Can you work these out from the model? Positions are in its coordinate system, mm. Face numbers are marked on the shaded views. A direction names the side the tool comes from. Round coordinates to 2 decimals unless told otherwise and drop trailing zeros. Loops run counter-clockwise (first coordinate to the right, second up) from the corner with the lowest first, then second, coordinate; pieces in that order, holes last. Notation, with made-up numbers: (47.5, 10.25) -> (66.5, 10.25) arc R22 ccw to (66.5, 44.25) -> close; hole circle Ø7 at (-22, 31). An arc over 180 degrees is marked (long way). Write item = value, one per line.
from build123d import *

# Parameters (mm, degrees)
F0_W     = 100
F0_H     = 100
F1_DEPTH = 50
F3_DEPTH = 100
F4_R     = 10
F5_DEPTH = 50
F7_DEPTH = 25
F8_W     = 80
F8_H     = 37.447
F9_DEPTH = 150


with BuildPart() as f1:
    # F0 (on Top) → F1 (new body)
    with BuildSketch(Plane.XY):
        with Locations((-7.640187, 1.520901)):
            Rectangle(F0_W, F0_H)
    extrude(amount=F1_DEPTH)

    # F2 (on face) → F3 (cut)
    with BuildSketch(Plane.XZ.offset(48.479099)):
        Polygon((0, 52.099957), (-27.144263, 52.099957), (-27.144263, 7.099957), (17.855737, 7.099957), (17.855737, 52.099957), align=None)
    extrude(amount=-F3_DEPTH, mode=Mode.SUBTRACT)

    # F4 (on face) → F5 (join)
    with BuildSketch(Plane(origin=(0, 0, 0), x_dir=(1, 0, 0), z_dir=(0, 0, -1))):
        with Locations((-57.640187, -51.520901)):
            Circle(F4_R)
        with Locations((-57.640187, 48.479099)):
            Circle(F4_R)
        with Locations((42.359813, 48.479099)):
            Circle(F4_R)
        with Locations((42.359813, -51.520901)):
            Circle(F4_R)
    extrude(amount=-F5_DEPTH)

    # F6 (on face) → F7 (cut)
    with BuildSketch(Plane(origin=(0, 0, 0), x_dir=(1, 0, 0), z_dir=(0, 0, -1))):
        Polygon((-14.585404, 10.162264), (-14.585404, -11.031568), (5.571128, -17.580822), (18.02855, -0.434652), (5.571128, 16.711519), align=None)
    extrude(amount=-F7_DEPTH, mode=Mode.SUBTRACT)

    # F8 (on face) → F9 (cut)
    with BuildSketch(Plane(origin=(-57.640187, 0, 0), x_dir=(0, -1, 0), z_dir=(-1, 0, 0))):
        with Locations((-1.520901, 31.2765)):
            Rectangle(F8_W, F8_H)
    extrude(amount=-F9_DEPTH, mode=Mode.SUBTRACT)


solid = f1.part
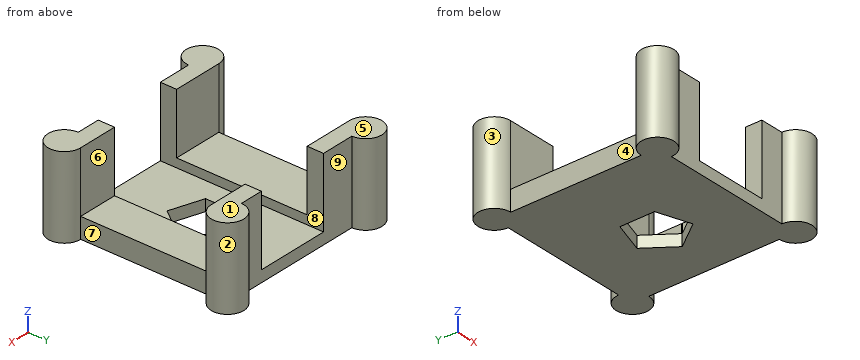
1. Suppose I cut it at A-A, the plane z = 10. List the corners of the cut face in (x, y) for me.
Entries:
outline = (-57.64, -38.48) arc R10 ccw (long way) to (-47.64, -48.48) -> (-27.14, -48.48) -> (-27.14, 51.52) -> (-47.64, 51.52) arc R10 ccw (long way) to (-57.64, 41.52) -> close; (17.86, -48.48) -> (32.36, -48.48) arc R10 ccw (long way) to (42.36, -38.48) -> (42.36, 41.52) arc R10 ccw (long way) to (32.36, 51.52) -> (17.86, 51.52) -> (17.86, 0.67) -> (18.03, 0.43) -> (17.86, 0.2) -> close
2. Suppose I cut it at D-D, the plane y = 38. List the corners of the cut face in (x, z) for me, and give its area (3 significant figures).
Entries:
outline = (-57.64, 0) -> (42.36, 0) -> (42.36, 12.55) -> (17.86, 12.55) -> (17.86, 7.1) -> (-27.14, 7.1) -> (-27.14, 12.55) -> (-57.64, 12.55) -> close
area = 1,010 mm²
3. We'd pull the mould along X, two halves only. Please class the marked faces 1, 2, 3 and 4: released by +X, released by -X, zero draft, split by the parting line, or undercut.
Entries:
face_1 = zero draft
face_2 = undercut
face_3 = undercut
face_4 = released by -X
4. For the marked faces 5, 6, 7, 8 and 9, which set-ups out of +Z, -Z, +X, -X, +Y, -Y let a thin tool reach every point of the face, with its end or its side?
Entries:
face_5 = +Z, +X, -X, +Y, -Y
face_6 = +Z, +X, -X
face_7 = +Z, -Z, +X
face_8 = +Z, +Y, -Y
face_9 = +Z, -Z, +Y
5. Suppose I cut it at B-B, the plane z = 17.5. List the corners of the cut face in (x, y) for me, and give its area (3 significant figures).
Entries:
outline = (-57.64, -38.48) arc R10 ccw (long way) to (-47.64, -48.48) -> (-27.14, -48.48) -> (-27.14, -38.48) -> close; (-57.64, 41.52) -> (-27.14, 41.52) -> (-27.14, 51.52) -> (-47.64, 51.52) arc R10 ccw (long way) to start; (17.86, -48.48) -> (32.36, -48.48) arc R10 ccw (long way) to (42.36, -38.48) -> (17.86, -38.48) -> close; (17.86, 41.52) -> (42.36, 41.52) arc R10 ccw (long way) to (32.36, 51.52) -> (17.86, 51.52) -> close
area = 2,040 mm²
6. I need wall thicknesses on line 1 (Y direction, x = -43.5, z = 38); line 2 (X direction, y = 37, z = 9.5); line 3 (Z direction, x = 12, y = -21.5). Which ranges of each line are inside material? Lowest first, please. Write a range as [from, to].
Entries:
line_1 = [-48.48, -38.48], [41.52, 51.52]
line_2 = [-57.64, -27.14], [17.86, 42.36]
line_3 = [0, 7.1]
7. I'm going to push flat-ended pins straight in: pin 1 (7.5 mm diameter, centred on x = 28, z = 27, fed in from +Y); pin 2 (15 mm diameter, centred on x = -21.5, z = 30.5, fed in from -Y); pin 3 (19.5 mm diameter, centred on x = 31, y = -11.5, fed in from +Z); pin 4 (6 mm diameter, centred on x = -22, z = 13, fed in from -Y). Where does each tip first touch, or does it pass through?
Entries:
pin_1 = 51.52
pin_2 = -48.48
pin_3 = 12.55
pin_4 = through
8. Suppose I cut it at C-C, the plane x = -44. List the corners of the cut face in (y, z) for me, and give its area (3 significant figures).
Entries:
outline = (-48.48, 0) -> (51.52, 0) -> (51.52, 50) -> (41.52, 50) -> (41.52, 12.55) -> (-38.48, 12.55) -> (-38.48, 50) -> (-48.48, 50) -> close
area = 2,000 mm²
